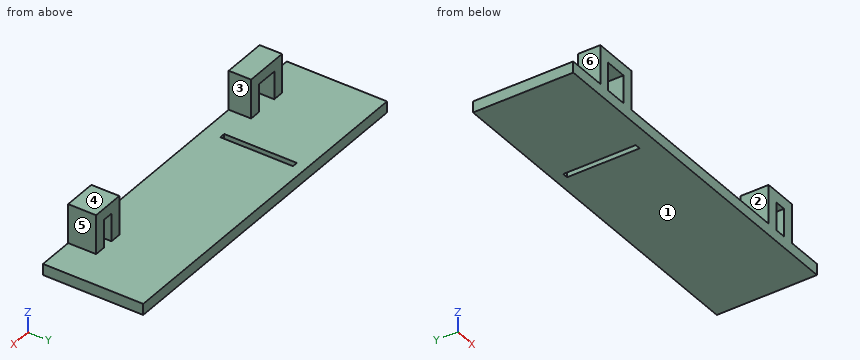
from build123d import *

# Parameters (mm, degrees)
P_IDAT_VYSUNUT_M1_DEPTH        = 2
SKICA3_R                       = 2.45
P_IDAT_VYSUNUT_M3_DEPTH        = 5
P_IDAT_VYSUNUT_M4_DEPTH        = 37.5
SKICA8_W                       = 10
SKICA8_H                       = 10
ODEBRAT_VYSUNUT_M2_DEPTH       = 4
SKICA10_W                      = 27.5
SKICA10_H                      = 79
ODEBRAT_VYSUNUT_M3_DEPTH       = 3
P_IDAT_VYSUNUT_M5_DEPTH        = 1
SKICA13_W                      = 3
SKICA13_H                      = 36.5
ODEBRAT_VYSUNUT_M6_DEPTH       = 103.45
SKICA14_W                      = 3
SKICA14_H                      = 36.5
ODEBRAT_VYSUNUT_M7_DEPTH       = 103.45
SKICA15_W                      = 36.5
SKICA15_H                      = 3
ODEBRAT_VYSUNUT_M8_DEPTH       = 61
SKICA19_W                      = 37
SKICA19_H                      = 13
ODEBRAT_VYSUNUT_M9_DEPTH       = 4
SKICA20_W                      = 63
SKICA20_H                      = 102.45
SKICA20_W_2                    = 57
SKICA20_H_2                    = 79
ODEBRAT_VYSUNUT_M10_DEPTH      = 1
SKICA22_W                      = 8
SKICA22_H                      = 4
SKICA22_W_2                    = 6
SKICA22_H_2                    = 5
P_IDAT_VYSUNUT_M6_DEPTH        = 7
SKICA23_W                      = 4
SKICA23_H                      = 5
SKICA23_W_2                    = 2
ODEBRAT_VYSUNUT_M12_DEPTH      = 5
SKICA25_W                      = 1
SKICA25_H                      = 13
ODEBRAT_VYSUNUT_M13_DEPTH      = 10
SKICA28_W                      = 63
SKICA28_H                      = 84.509642994
ODEBRAT_VYSUNUT_M14_DEPTH      = 8
ODEBRAT_VYSUNUT_M14_DEPTH_BACK = 3


with BuildPart() as part:
    # Skica1 → Přidat vysunutím1 (new body)
    with BuildSketch(Plane.XY):
        Polygon((13, -102.45), (13, -115.45), (50, -115.45), (50, -102.45), (63, -102.45), (63, 0), (0, 0), (0, -102.45), align=None)
    extrude(amount=P_IDAT_VYSUNUT_M1_DEPTH)

    # Skica3 → Přidat vysunutím3 (add)
    with BuildSketch(Plane.XY.offset(2)):
        with Locations((7.55, -6.45)):
            Circle(SKICA3_R)
        with Locations((7.55, -78.45)):
            Circle(SKICA3_R)
        with Locations((55.55, -78.45)):
            Circle(SKICA3_R)
        with Locations((55.55, -6.45)):
            Circle(SKICA3_R)
    extrude(amount=P_IDAT_VYSUNUT_M3_DEPTH)

    # Skica4 → Přidat vysunutím4 (add)
    with BuildSketch(Plane.XY.offset(2)):
        Polygon((63, 0), (63, -102.45), (60, -102.45), (60, -3), (3, -3), (3, -102.45), (0, -102.45), (0, 0), align=None)
    extrude(amount=P_IDAT_VYSUNUT_M4_DEPTH)

    # Skica8 → Odebrat vysunutím2 (cut, through all)
    with BuildSketch(Plane.ZY.offset(-60)):
        with Locations((7, -49)):
            Rectangle(SKICA8_W, SKICA8_H)
    extrude(amount=-ODEBRAT_VYSUNUT_M2_DEPTH, mode=Mode.SUBTRACT)

    # Skica10 → Odebrat vysunutím3 (cut)
    with BuildSketch(Plane.ZY):
        with Locations((25.75, -42.5)):
            Rectangle(SKICA10_W, SKICA10_H)
    extrude(amount=-ODEBRAT_VYSUNUT_M3_DEPTH, mode=Mode.SUBTRACT)

    # Skica11 → Přidat vysunutím5 (add)
    with BuildSketch(Plane.XY.offset(2)):
        Polygon((3, -82), (60, -82), (60, -102.45), (50, -102.45), (50, -115.45), (13, -115.45), (13, -102.45), (3, -102.45), align=None)
    extrude(amount=P_IDAT_VYSUNUT_M5_DEPTH)

    # Skica13 → Odebrat vysunutím6 (cut, through all)
    with BuildSketch(Plane.XZ.offset(102.45)):
        with Locations((1.5, 21.25)):
            Rectangle(SKICA13_W, SKICA13_H)
    extrude(amount=-ODEBRAT_VYSUNUT_M6_DEPTH, mode=Mode.SUBTRACT)

    # Skica14 → Odebrat vysunutím7 (cut, through all)
    with BuildSketch(Plane.XZ.offset(102.45)):
        with Locations((61.5, 21.25)):
            Rectangle(SKICA14_W, SKICA14_H)
    extrude(amount=-ODEBRAT_VYSUNUT_M7_DEPTH, mode=Mode.SUBTRACT)

    # Skica15 → Odebrat vysunutím8 (cut, through all)
    with BuildSketch(Plane.ZY.offset(-3)):
        with Locations((21.25, -1.5)):
            Rectangle(SKICA15_W, SKICA15_H)
    extrude(amount=-ODEBRAT_VYSUNUT_M8_DEPTH, mode=Mode.SUBTRACT)

    # Skica19 → Odebrat vysunutím9 (cut, through all)
    with BuildSketch(Plane.XY.offset(3)):
        with Locations((31.5, -108.95)):
            Rectangle(SKICA19_W, SKICA19_H)
    extrude(amount=-ODEBRAT_VYSUNUT_M9_DEPTH, mode=Mode.SUBTRACT)

    # Skica20 → Odebrat vysunutím10 (cut)
    with BuildSketch(Plane.XY.offset(3)):
        with Locations((31.5, -51.225)):
            Rectangle(SKICA20_W, SKICA20_H)
        with Locations((31.5, -42.5)):
            Rectangle(SKICA20_W_2, SKICA20_H_2, mode=Mode.SUBTRACT)
    extrude(amount=-ODEBRAT_VYSUNUT_M10_DEPTH, mode=Mode.SUBTRACT)

    # Skica22 → Přidat vysunutím6 (add)
    with BuildSketch(Plane.XY.offset(2)):
        with Locations((11, -100.45)):
            Rectangle(SKICA22_W, SKICA22_H)
        with Locations((53.5, -99.95)):
            Rectangle(SKICA22_W_2, SKICA22_H_2)
    extrude(amount=P_IDAT_VYSUNUT_M6_DEPTH)

    # Skica23 → Odebrat vysunutím12 (cut)
    with BuildSketch(Plane.XZ.offset(102.45)):
        with Locations((11, 4.5)):
            Rectangle(SKICA23_W, SKICA23_H)
        with Locations((53.5, 4.5)):
            Rectangle(SKICA23_W_2, SKICA23_H)
    extrude(amount=-ODEBRAT_VYSUNUT_M12_DEPTH, mode=Mode.SUBTRACT)

    # Skica25 → Odebrat vysunutím13 (cut)
    with BuildSketch(Plane.XY.offset(2)):
        with Locations((21, -92.95)):
            Rectangle(SKICA25_W, SKICA25_H)
    extrude(amount=-ODEBRAT_VYSUNUT_M13_DEPTH, mode=Mode.SUBTRACT)

    # Skica28 → Odebrat vysunutím14 (cut, two sides)
    with BuildSketch(Plane.XY.offset(2)) as odebrat_vysunut_m14_sk:
        with Locations((31.5, -42.254821497)):
            Rectangle(SKICA28_W, SKICA28_H)
    extrude(amount=ODEBRAT_VYSUNUT_M14_DEPTH, mode=Mode.SUBTRACT)
    extrude(odebrat_vysunut_m14_sk.sketch, amount=-ODEBRAT_VYSUNUT_M14_DEPTH_BACK, mode=Mode.SUBTRACT)


solid = part.part
The listing builds one solid part. Answer for the finished solid, in the listing's coordinates (mm). Face numbers are marked on the shaded views. A direction names the side the tool comes from. Give positions to 0.01 mm unless a question says otherwise; leave off trailing zeros. Order: outer loops, then holes, each group sorted by start corner. A loop starts at its lowest first (then second) coordinate and runs counter-clockwise, first axis right, second up. Notation, with made-up numbers: (-6.75, 58.25) - (43.25, 58.25) arc R20 cw to (43.25, 62.25) - close; hole circle Ø7 at (84, 45). An arc over 180 degrees is marked (long way). Use one line per item in the form item = value.
1) Find section D-D on z = 4. Determine the outline of the cut face in (x, y).
Verdict:
outline = (7, -102.45) - (9, -102.45) - (9, -98.45) - (7, -98.45) - close; (13, -102.45) - (15, -102.45) - (15, -98.45) - (13, -98.45) - close; (50.5, -102.45) - (52.5, -102.45) - (52.5, -97.45) - (50.5, -97.45) - close; (54.5, -102.45) - (56.5, -102.45) - (56.5, -97.45) - (54.5, -97.45) - close
2) Find section B-B on x = 53.5. Determine the outline of the cut face in (y, z), and give its area (3 significant figures).
Verdict:
outline = (-102.45, 0) - (-84.51, 0) - (-84.51, 2) - (-102.45, 2) - close; (-102.45, 7) - (-97.45, 7) - (-97.45, 9) - (-102.45, 9) - close
area = 45.9 mm^2
3) Consider probe 1 along X at (y, z) = (-100, 6.5); probe 2 along X at (y, z) = (-99, 1.5); probe 3 along X at (y, z) = (-97.75, 5). Determine where each line is inside the solid, lowest interval first. Write a range as [from, to].
Verdict:
probe_1 = [7, 9], [13, 15], [50.5, 52.5], [54.5, 56.5]
probe_2 = [0, 20.5], [21.5, 63]
probe_3 = [50.5, 52.5], [54.5, 56.5]
4) The mould has two halves that part along X. Classify the marked faces 3, 4, 5 and 6: released by +X, released by -X, zero draft, split by the parting line, or undercut.
Verdict:
face_3 = undercut
face_4 = zero draft
face_5 = released by +X
face_6 = released by -X
5) Each of these flat-tipped pins is pushed along its axis until it touches: pin 1 (1 mm diameter, centred on y = -99.5, z = 4, fed in from +X); pin 2 (4 mm diameter, centred on x = 28, y = -96, fed in from +Z); pin 3 (1 mm diameter, centred on x = 45.5, z = 3.5, fed in from -Y); pin 4 (2.5 mm diameter, centred on y = -100, z = 5.5, fed in from -X). Where does it stop, or does it pass through?
Verdict:
pin_1 = 56.5
pin_2 = 2
pin_3 = through
pin_4 = 7
6) Find section A-A on y = -95. Determine the outline of the cut face in (x, z), and give its area (3 significant figures).
Verdict:
outline = (0, 0) - (20.5, 0) - (20.5, 2) - (0, 2) - close; (21.5, 0) - (63, 0) - (63, 2) - (21.5, 2) - close
area = 124 mm^2
7) Find section C-C on y = -100.5. Determine the outline of the cut face in (x, z).
Verdict:
outline = (0, 0) - (63, 0) - (63, 2) - (56.5, 2) - (56.5, 9) - (50.5, 9) - (50.5, 2) - (15, 2) - (15, 9) - (7, 9) - (7, 2) - (0, 2) - close; hole (9, 2) - (13, 2) - (13, 7) - (9, 7) - close; hole (52.5, 2) - (54.5, 2) - (54.5, 7) - (52.5, 7) - close
8) For the marked faces 1 and 2, determine the directions among +Z, -Z, +X, -X, +Y, -Y from which every point of the face is accessible in a straight line to the end or side of a thin tool.
Verdict:
face_1 = -Z, +X, -X, +Y, -Y
face_2 = +Z, +Y, -Y
